Read the model definition and answer for the solid it produces. Units are mm, in the model's axes. Face numbers are marked on the shaded views. A direction names the side the tool comes from. Coordinates: 2 decimals unless noted, no trailing zeros. Write each loop counter-clockwise with the first axis right and the second up, starting at its lowest first coordinate (ties: lowest second). Pieces come first, ordered by that corner, then holes.
1) Which of the six approach directions +Z, -Z, +X, -X, +Y, -Y give full straight-line access (tool end or side, diameter ignored) to the marked faces 1, 2, 3 and 4?
2) The part is cut by section C-C (x = 27.25). Determine the outline of the cut face in (y, z), then the cut area to 3 significant figures.
3) Each of these flat-tipped pins is pushed along its axis until it touches: pin 1 Ø3 at (x, y) = (31.26, -3.85) entering from +Z; pin 2 Ø6 at (y, z) = (-6, 9.5) entering from +X; pin 3 Ø3 at (x, y) = (30.5, -4.5) entering from +Z; pin 4 Ø1.7 at (x, y) = (32.5, -5) entering from -Z. Where does it stop, or does it pass through?
4) The part is cut by section B-B (x = 22.25). Determine the outline of the cut face in (y, z).
5) The part is cut by section A-A (z = -4). Determine the outline of the cut face in (x, y), then the cut area to 3 significant figures.
6) The part is cut by section D-D (y = -0.5). Determine the outline of the cut face in (x, z), then the cut area to 3 significant figures.
7) Find the intervals of material crossed by line 1 (Z direction, x = 18.75, y = -3); line 2 (Y direction, x = 22, z = -10); line 3 (X direction, y = -3.75, z = 7.5), in increasing order.
from build123d import *

# Parameters (mm, degrees)
SKETCH1_W           = 27.6
SKETCH1_H           = 30.9
BOSS_EXTRUDE1_DEPTH = 2
SKETCH2_W           = 20.2
SKETCH2_H           = 27.3
BOSS_EXTRUDE2_DEPTH = 8
SKETCH3_R           = 1.6
CUT_EXTRUDE1_DEPTH  = 32
CUT_EXTRUDE2_DEPTH  = 2.5
CUT_EXTRUDE3_DEPTH  = 2.5


with BuildPart() as part:
    # Sketch1 → Boss-Extrude1 (new body)
    with BuildSketch(Plane(origin=(0, 0, 0), x_dir=(1, 0, 0), z_dir=(0, 1, 0))):
        with Locations((25.658887851, 1.636558914)):
            Rectangle(SKETCH1_W, SKETCH1_H)
    extrude(amount=BOSS_EXTRUDE1_DEPTH)

    # Sketch2 → Boss-Extrude2 (add)
    with BuildSketch(Plane.XZ):
        with Locations((26.058887851, 0.163441086)):
            Rectangle(SKETCH2_W, SKETCH2_H)
    extrude(amount=BOSS_EXTRUDE2_DEPTH)

    # Sketch3 → Cut-Extrude1 (cut)
    with BuildSketch(Plane.XY.offset(13.813441086)):
        with Locations((21.258887851, -3.85)):
            Circle(SKETCH3_R)
        with Locations((31.258887851, -3.85)):
            Circle(SKETCH3_R)
    extrude(amount=-CUT_EXTRUDE1_DEPTH, mode=Mode.SUBTRACT)

    # Sketch4 → Cut-Extrude2 (cut)
    with BuildSketch(Plane.XY.offset(12.313441086)):
        Polygon((32.875468605, -6.65), (34.492049359, -3.85), (32.875468605, -1.05), (29.642307097, -1.05), (28.025726344, -3.85), (29.642307097, -6.65), align=None)
        Polygon((22.91999145, -6.623818337), (24.491636796, -3.798351254), (22.830533197, -1.024532917), (19.597784252, -1.076181663), (18.026138906, -3.901648746), (19.687242505, -6.675467083), align=None)
    extrude(amount=-CUT_EXTRUDE2_DEPTH, mode=Mode.SUBTRACT)

    # Sketch5 → Cut-Extrude3 (cut)
    with BuildSketch(Plane(origin=(0, 0, -11.986558914), x_dir=(-1, 0, 0), z_dir=(0, 0, -1))):
        Polygon((-29.642307097, -6.65), (-28.025726344, -3.85), (-29.642307097, -1.05), (-32.875468605, -1.05), (-34.492049359, -3.85), (-32.875468605, -6.65), align=None)
        Polygon((-19.642307097, -6.65), (-18.025726344, -3.85), (-19.642307097, -1.05), (-22.875468605, -1.05), (-24.492049359, -3.85), (-22.875468605, -6.65), align=None)
    extrude(amount=-CUT_EXTRUDE3_DEPTH, mode=Mode.SUBTRACT)


solid = part.part
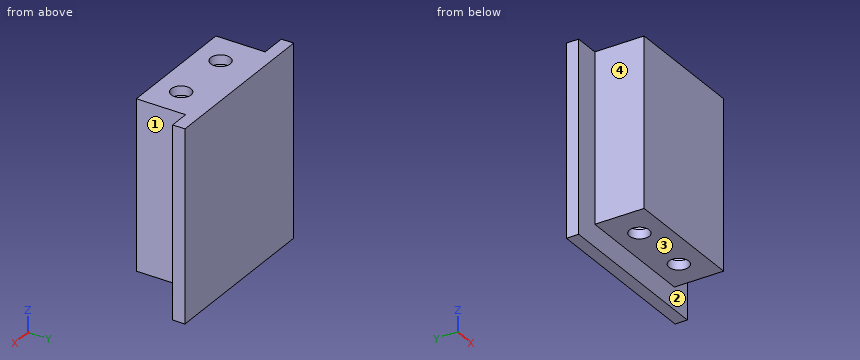
Reported:
1. face 1: +Z, -Z, +X, -Y
1. face 2: -Z, -Y
1. face 3: -Z, +X, -X, -Y
1. face 4: +Z, -Z, -X, -Y
2. outline: (-8, -13.49) - (0, -13.49) - (0, -17.09) - (2, -17.09) - (2, 13.81) - (-8, 13.81) - close
2. area: 280 mm2
3. pin 1: passes through
3. pin 2: stops at x = 36.16
3. pin 3: stops at z = 13.81
3. pin 4: stops at z = -13.49
4. outline: (-8, -13.49) - (-5.11, -13.49) - (-5.11, -11.99) - (-6.65, -11.99) - (-6.65, -9.49) - (-5.11, -9.49) - (-5.11, 9.81) - (-6.63, 9.81) - (-6.63, 12.31) - (-5.11, 12.31) - (-5.11, 13.81) - (-8, 13.81) - close; (-2.59, -13.49) - (0, -13.49) - (0, -17.09) - (2, -17.09) - (2, 13.81) - (-2.59, 13.81) - (-2.59, 12.31) - (-1.03, 12.31) - (-1.03, 9.81) - (-2.59, 9.81) - (-2.59, -9.49) - (-1.05, -9.49) - (-1.05, -11.99) - (-2.59, -11.99) - close
5. outline: (11.86, 0) - (15.96, 0) - (15.96, -8) - (36.16, -8) - (36.16, 0) - (39.46, 0) - (39.46, 2) - (11.86, 2) - close; hole circle Ø3.2 at (21.26, -3.85); hole circle Ø3.2 at (31.26, -3.85)
5. area: 201 mm2
6. outline: (15.96, -13.49) - (36.16, -13.49) - (36.16, 13.81) - (15.96, 13.81) - close
6. area: 551 mm2
7. line 1: z = -13.49 to -11.99, -9.49 to 9.81, 12.31 to 13.81
7. line 2: y = -8 to -6.65, -1.05 to 2
7. line 3: x = 15.96 to 19.66, 22.86 to 29.66, 32.86 to 36.16
